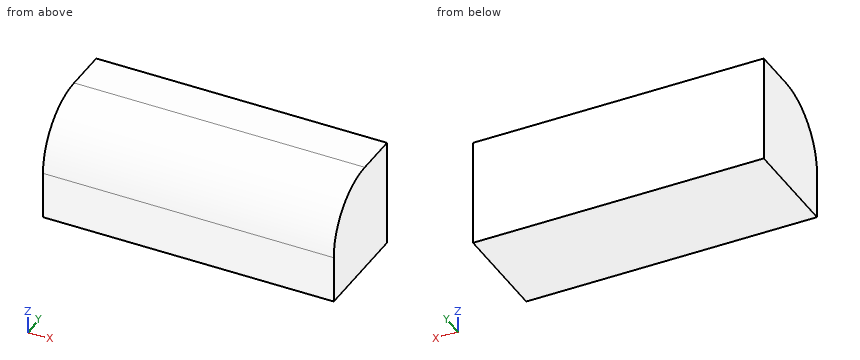
```python
from build123d import *

# Parameters (mm, degrees)
SKETCH1_W            = 48
SKETCH1_H            = 53
BOSS_EXTRUDE1_DEPTH  = 10
SKETCH2_W            = 48
SKETCH2_H            = 5.616325
BOSS_EXTRUDE2_DEPTH  = 33.1917878
SKETCH4_W            = 4
SKETCH4_H            = 10
BOSS_EXTRUDE4_DEPTH  = 40
SKETCH5_W            = 48
SKETCH5_H            = 10.8609375
BOSS_EXTRUDE5_DEPTH  = 23.1917878
SKETCH6_W            = 48
SKETCH6_H            = 5
BOSS_EXTRUDE6_DEPTH  = 42.3
SKETCH7_W            = 12.8082122
SKETCH7_H            = 16.4772625
BOSS_EXTRUDE7_DEPTH  = 48
CUT_EXTRUDE1_REACH   = 84.426
SKETCH8_R            = 11.5
SKETCH8_R_2          = 2
FILLET1_R            = 10
FILLET2_R            = 4
SKETCH9_W            = 5
SKETCH9_H            = 16.4772625
BOSS_EXTRUDE9_DEPTH  = 48
CUT_EXTRUDE2_DEPTH   = 6
SKETCH11_R           = 1.9304
CUT_EXTRUDE3_DEPTH   = 6
BOSS_EXTRUDE11_DEPTH = 3
BOSS_EXTRUDE12_DEPTH = 48
SKETCH14_W           = 119.824941969
SKETCH14_H           = 122.237524693
CUT_EXTRUDE4_DEPTH   = 90.10667764


with BuildPart() as part:
    # Sketch1 → Boss-Extrude1 (new body)
    with BuildSketch(Plane.XY):
        with Locations((24, 26.5)):
            Rectangle(SKETCH1_W, SKETCH1_H)
    extrude(amount=BOSS_EXTRUDE1_DEPTH)

    # Sketch2 → Boss-Extrude2 (add)
    with BuildSketch(Plane(origin=(0, 0, 0), x_dir=(-1, 0, 0), z_dir=(0, 0, -1))):
        with Locations((-24, -2.8081625)):
            Rectangle(SKETCH2_W, SKETCH2_H)
    extrude(amount=-BOSS_EXTRUDE2_DEPTH)

    # Sketch4 → Boss-Extrude4 (add)
    with BuildSketch(Plane.XY.offset(10)):
        with Locations((2, 48)):
            Rectangle(SKETCH4_W, SKETCH4_H)
        with Locations((46, 48)):
            Rectangle(SKETCH4_W, SKETCH4_H)
    extrude(amount=BOSS_EXTRUDE4_DEPTH)

    # Sketch5 → Boss-Extrude5 (add)
    with BuildSketch(Plane.XY.offset(10)):
        with Locations((24, 5.43046875)):
            Rectangle(SKETCH5_W, SKETCH5_H)
    extrude(amount=BOSS_EXTRUDE5_DEPTH)

    # Sketch6 → Boss-Extrude6 (add)
    with BuildSketch(Plane.XZ.offset(5.616325)):
        with Locations((24, 30.6917878)):
            Rectangle(SKETCH6_W, SKETCH6_H)
    extrude(amount=BOSS_EXTRUDE6_DEPTH)

    # Sketch7 → Boss-Extrude7 (add)
    with BuildSketch(Plane.ZY):
        with Locations((-6.4041061, 2.62230625)):
            Rectangle(SKETCH7_W, SKETCH7_H)
    extrude(amount=-BOSS_EXTRUDE7_DEPTH)

    # Sketch8 → Cut-Extrude1 (cut, up to next)
    with BuildSketch(Plane(origin=(0, 0, 28.1917878), x_dir=(-1, 0, 0), z_dir=(0, 0, -1)), mode=Mode.PRIVATE) as cut_extrude1_sk1:
        with Locations((-24, -26.616325)):
            Circle(SKETCH8_R)
    cut_extrude1_tool1 = extrude(cut_extrude1_sk1.sketch, amount=-CUT_EXTRUDE1_REACH, mode=Mode.PRIVATE) & part.part
    # Sketch8 → Cut-Extrude1 (cut, up to next)
    with BuildSketch(Plane(origin=(0, 0, 28.1917878), x_dir=(-1, 0, 0), z_dir=(0, 0, -1)), mode=Mode.PRIVATE) as cut_extrude1_sk2:
        with Locations((-39.5, -11.116325)):
            Circle(SKETCH8_R_2)
    cut_extrude1_tool2 = extrude(cut_extrude1_sk2.sketch, amount=-CUT_EXTRUDE1_REACH, mode=Mode.PRIVATE) & part.part
    # Sketch8 → Cut-Extrude1 (cut, up to next)
    with BuildSketch(Plane(origin=(0, 0, 28.1917878), x_dir=(-1, 0, 0), z_dir=(0, 0, -1)), mode=Mode.PRIVATE) as cut_extrude1_sk3:
        with Locations((-39.5, -42.116325)):
            Circle(SKETCH8_R_2)
    cut_extrude1_tool3 = extrude(cut_extrude1_sk3.sketch, amount=-CUT_EXTRUDE1_REACH, mode=Mode.PRIVATE) & part.part
    # Sketch8 → Cut-Extrude1 (cut, up to next)
    with BuildSketch(Plane(origin=(0, 0, 28.1917878), x_dir=(-1, 0, 0), z_dir=(0, 0, -1)), mode=Mode.PRIVATE) as cut_extrude1_sk4:
        with Locations((-8.5, -11.116325)):
            Circle(SKETCH8_R_2)
    cut_extrude1_tool4 = extrude(cut_extrude1_sk4.sketch, amount=-CUT_EXTRUDE1_REACH, mode=Mode.PRIVATE) & part.part
    # Sketch8 → Cut-Extrude1 (cut, up to next)
    with BuildSketch(Plane(origin=(0, 0, 28.1917878), x_dir=(-1, 0, 0), z_dir=(0, 0, -1)), mode=Mode.PRIVATE) as cut_extrude1_sk5:
        with Locations((-8.5, -42.116325)):
            Circle(SKETCH8_R_2)
    cut_extrude1_tool5 = extrude(cut_extrude1_sk5.sketch, amount=-CUT_EXTRUDE1_REACH, mode=Mode.PRIVATE) & part.part
    add(cut_extrude1_tool1.solids().sort_by_distance((24, -26.616325, 28.191788))[0], mode=Mode.SUBTRACT)
    add(cut_extrude1_tool2.solids().sort_by_distance((39.5, -11.116325, 28.191788))[0], mode=Mode.SUBTRACT)
    add(cut_extrude1_tool3.solids().sort_by_distance((39.5, -42.116325, 28.191788))[0], mode=Mode.SUBTRACT)
    add(cut_extrude1_tool4.solids().sort_by_distance((8.5, -11.116325, 28.191788))[0], mode=Mode.SUBTRACT)
    add(cut_extrude1_tool5.solids().sort_by_distance((8.5, -42.116325, 28.191788))[0], mode=Mode.SUBTRACT)

    # Fillet1
    fillet1_edges = [part.edges().sort_by_distance(p)[0] for p in [
        (24, 10.8609375, 0),
    ]]
    fillet(fillet1_edges, radius=FILLET1_R)

    # Fillet2
    fillet2_edges = [part.edges().sort_by_distance(p)[0] for p in [
        (2, 43, 10),
        (46, 43, 10),
    ]]
    fillet(fillet2_edges, radius=FILLET2_R)

    # Sketch9 → Boss-Extrude9 (add)
    with BuildSketch(Plane(origin=(48, 0, 0), x_dir=(0, 0, -1), z_dir=(1, 0, 0))):
        with Locations((15.3082122, 2.62230625)):
            Rectangle(SKETCH9_W, SKETCH9_H)
    extrude(amount=-BOSS_EXTRUDE9_DEPTH)

    # Sketch10 → Cut-Extrude2 (cut)
    with BuildSketch(Plane.XY.offset(10)):
        Polygon((12.429, 36.979734073), (9, 38.959468146), (5.571, 36.979734073), (5.571, 33.020265927), (9, 31.040531854), (12.429, 33.020265927), align=None)
        Polygon((35.571, 36.979734073), (35.571, 33.020265927), (39, 31.040531854), (42.429, 33.020265927), (42.429, 36.979734073), (39, 38.959468146), align=None)
    extrude(amount=-CUT_EXTRUDE2_DEPTH, mode=Mode.SUBTRACT)

    # Sketch11 → Cut-Extrude3 (cut)
    with BuildSketch(Plane.XY.offset(4)):
        with Locations((9, 35)):
            Circle(SKETCH11_R)
        with Locations((39, 35)):
            Circle(SKETCH11_R)
    extrude(amount=-CUT_EXTRUDE3_DEPTH, mode=Mode.SUBTRACT)

    # Sketch12 → Boss-Extrude11 (add)
    with BuildSketch(Plane(origin=(0, 53, 0), x_dir=(1, 0, 0), z_dir=(0, 1, 0))):
        Polygon((0, 0), (0, -50), (4, -50), (4, -10), (44, -10), (44, -50), (48, -50), (48, 0), align=None)
    extrude(amount=BOSS_EXTRUDE11_DEPTH)

    # Sketch13 → Boss-Extrude12 (add)
    with BuildSketch(Plane(origin=(48, 0, 0), x_dir=(0, 0, -1), z_dir=(1, 0, 0))):
        with BuildLine():
            Line((17.8082122, 10.8609375), (10, 10.8609375))
            ThreePointArc((10, 10.8609375), (2.928932188, 13.789869688), (0, 20.8609375))
            Line((0, 20.8609375), (0, 28))
            Line((0, 28), (17.8082122, 28))
            Line((17.8082122, 28), (17.8082122, 10.8609375))
        make_face()
    extrude(amount=-BOSS_EXTRUDE12_DEPTH)

    # Sketch14 → Cut-Extrude4 (cut, through all)
    with BuildSketch(Plane(origin=(48, 0, 0), x_dir=(0, 0, -1), z_dir=(1, 0, 0))):
        with Locations((-16.90365686, 8.216937598)):
            Rectangle(SKETCH14_W, SKETCH14_H)
        with BuildLine():
            Line((0, 28), (0, 20.8609375))
            ThreePointArc((0, 20.8609375), (2.928932188, 13.789869688), (10, 10.8609375))
            Line((10, 10.8609375), (17.8082122, 10.8609375))
            Line((17.8082122, 10.8609375), (17.8082122, 28))
            Line((17.8082122, 28), (0, 28))
        make_face(mode=Mode.SUBTRACT)
    extrude(amount=-CUT_EXTRUDE4_DEPTH, mode=Mode.SUBTRACT)


solid = part.part
```
Read the model definition and answer for the solid it produces. Units are mm, in the model's axes. Give positions to 0.01 mm unless a question says otherwise; leave off trailing zeros. Write each loop counter-clockwise with the first axis right and the second up, starting at its lowest first coordinate (ties: lowest second). Pieces come first, ordered by that corner, then holes. Notation, with made-up numbers: M -17,2.5 L 9,2.5 A20 ccw 9,16.5 Z; hole C -37.5,70.5 d7. An arc over 180 degrees is marked long. Put each result on its own line as item: value. Start each with the question number.
1. The part is cut by section C-C, the plane z = -2. Give the vertices of the cut face in (x, y), and give its area (3 significant figures).
2. Consider line 1 along Z through (x, y) = (46, 16.25); line 2 along Y through (x, z) = (31, -6.25); line 3 along Z through (x, y) = (5.5, 12). Determine where each line is inside the solid, lowest interval first.
3. The part is cut by section A-A, the plane x = 39.5. Give the vertices of the cut face in (y, z).
4. This flat-tipped pin is pushed along its axis until it touches: pin 1 Ø1.5 at (x, z) = (9, -7) entering from -Y. Where does it stop, or does it pass through?
5. The part is cut by section B-B, the plane y = 13.75. Give the vertices of the cut face in (x, z).
Final values:
1. outline: M 0,14.86 L 48,14.86 L 48,28 L 0,28 Z
1. area: 631 mm²
2. line 1: z = -17.81 to -1.13
2. line 2: y = 11.59 to 28
2. line 3: z = -17.81 to -5.36
3. outline: M 10.86,-17.81 L 28,-17.81 L 28,0 L 20.86,0 A10 ccw 10.86,-10 Z
4. pin 1: stops at y = 11.12
5. outline: M 0,-17.81 L 48,-17.81 L 48,-2.97 L 0,-2.97 Z
